Autodesk Inventor part; units mm, degrees
ref_plane "YZ Plane" through (0, 0, 0) normal (1, 0, 0) x (0, 1, 0)
ref_plane "XZ Plane" through (0, 0, 0) normal (0, 1, 0) x (-1, 0, 0)
ref_plane "XY Plane" through (0, 0, 0) normal (0, 0, 1) x (1, 0, 0)
sketch "Эскиз1" plane through (0, 0, 0) normal (0, 1, 0) x (-1, 0, 0)
  line L0 (35, 15.6528) -> (35, -5.6528)
  line L1 (-25, -5) -> (-25, 15)
  line L2 (30.6678, 19.639) -> (-25, 15)
  line L3 (30.6678, -9.639) -> (-25, -5)
  circle A0 centre (2.3404, 5) radius 2
  circle A1 centre (14.4404, 5) radius 3
  circle A2 centre (26.5404, 5) radius 2
  arc A3 (35, 15.6528) -> (30.6678, 19.639) centre (31, 15.6528) ccw
  arc A4 (30.6678, -9.639) -> (35, -5.6528) centre (31, -5.6528) ccw
  point P0 (0, 0)
  point P1 (35, -10)
  point P2 (35, 20)
  point P3 (12.9676, -25.8489)
  dimension "d0" = 30
  dimension "d4" = 60
  dimension "d6" = 15
  dimension "d8" = 4
extrude "Выдавливание1" add sketch "Эскиз1" along normal blind 10
properties part number "хуйня резня"
The model under review builds one solid part; all positions refer to its coordinate system, in mm. Coordinates: 2 decimals unless noted, no trailing zeros. Write each loop counter-clockwise with the first axis right and the second up, starting at its lowest first coordinate (ties: lowest second). Pieces come first, ordered by that corner, then holes. Notation, with made-up numbers: (5.5, 22) -> (38.5, 22) arc R24 ccw to (38.5, 52) -> close; hole circle Ø6 at (-39, -32.5). An arc over 180 degrees is marked (long way). One line per item, written item: value. Start each with the question number.
Q1. To check wall thickness, follow probe 1 along X at (y, z) = (1.25, 4.5); probe 2 along Z at (x, y) = (-1, 5.5); probe 3 along Z at (x, y) = (-25, 6.5). State the ranges of each line that lie inside material, in increasing order.
Q2. Add section C-C, the plane x = 6. Give the boundary of the cut face in (y, z).
Q3. Add section A-A, the plane z = 5. Give the boundary of the cut face in (x, y).
Q4. Add section D-D, the plane z = -6.75. Give the boundary of the cut face in (x, y).
Q5. Clearance check with flat-ended pins moving along their axes: P1, Ø3, axis at x = -4.5, y = 7.5, coming from the -Z side; P2, Ø1, axis at x = 11.5, y = 5, coming from the +Z side; P3, Ø1, axis at x = 5.5, y = 8, coming from the +Z side. State where each tip first meets the part, or that it passes through.
Q6. Add section B-B, the plane y = 6. Give the boundary of the cut face in (x, z), then the cut area to 3 significant figures.
Q7. The part is to be moulded in two halves that separate along Z. For faces 1 (the face through (-3.22, 4.93, 17.35)), 2 (the face through (-33.742, 4.93, -8.565)), 3 (the face through (-24.953, 4.93, 6.217)), say which applies: +Z half, -Z half, draft (parallel to the pull), parting line (faces both ways), or undercut.
Response:
1. probe 1: -35 to -28.48, -24.6 to -17.4, -11.48 to -4.28, -0.4 to 25
1. probe 2: -7.17 to 3.52, 6.48 to 17.17
1. probe 3: -9.17 to 3.72, 6.28 to 19.17
2. outline: (0, -6.58) -> (10, -6.58) -> (10, 16.58) -> (0, 16.58) -> close
3. outline: (-35, 0) -> (-28.54, 0) -> (-28.54, 10) -> (-35, 10) -> close; (-24.54, 0) -> (-17.44, 0) -> (-17.44, 10) -> (-24.54, 10) -> close; (-11.44, 0) -> (-4.34, 0) -> (-4.34, 10) -> (-11.44, 10) -> close; (-0.34, 0) -> (25, 0) -> (25, 10) -> (-0.34, 10) -> close
4. outline: (-34.85, 0) -> (4, 0) -> (4, 10) -> (-34.85, 10) -> close
5. P1: z = -7.58
5. P2: z = 16.17
5. P3: z = 16.67
6. outline: (-35, -5.65) arc R4 ccw to (-30.67, -9.64) -> (25, -5) -> (25, 15) -> (-30.67, 19.64) arc R4 ccw to (-35, 15.65) -> close; hole circle Ø4 at (-26.54, 5); hole circle Ø6 at (-14.44, 5); hole circle Ø4 at (-2.34, 5)
6. area: 1,440 mm²
7. face 1: +Z half
7. face 2: -Z half
7. face 3: undercut
